Read the model definition and answer for the solid it produces. Units are mm, in the model's axes. Face numbers are marked on the shaded views. A direction names the side the tool comes from. Coordinates: 2 decimals unless noted, no trailing zeros. Loops run counter-clockwise (first coordinate to the right, second up) from the corner with the lowest first, then second, coordinate; pieces in that order, holes last. Notation, with made-up numbers: M -3.75,-20.5 L 37.25,-20.5 A34 cw 37.25,16.5 Z; hole C -1,-33.5 d7. An arc over 180 degrees is marked long. Put each result on its own line as item: value.
from build123d import *
from OCP.BRepFilletAPI import BRepFilletAPI_MakeChamfer

# Parameters (mm, degrees)
BOSS_EXTRUDE1_DEPTH = 15
CHAMFER1_SIZE       = 15
CHAMFER1_SIZE2      = 2
SKETCH2_R           = 3
CUT_EXTRUDE1_DEPTH  = 15
CHAMFER2_SIZE       = 2


with BuildPart() as part:
    # Sketch1 → Boss-Extrude1 (new body)
    with BuildSketch(Plane(origin=(0, 0, 0), x_dir=(1, 0, 0), z_dir=(0, 1, 0))):
        with BuildLine():
            ThreePointArc((-10, 0), (0, 10), (10, 0))
            Line((10, 0), (10, 25))
            Line((10, 25), (-10, 25))
            Line((-10, 25), (-10, 0))
        make_face()
        with BuildLine():
            ThreePointArc((-4.8, 0), (0, 4.8), (4.8, 0))
            Line((4.8, 0), (10, 0))
            ThreePointArc((10, 0), (0, 10), (-10, 0))
            Line((-10, 0), (-4.8, 0))
        make_face()
        with BuildLine():
            Line((10, 0), (4.8, 0))
            ThreePointArc((4.8, 0), (0, -4.8), (-4.8, 0))
            Line((-4.8, 0), (-10, 0))
            ThreePointArc((-10, 0), (0, -10), (10, 0))
        make_face()
    extrude(amount=BOSS_EXTRUDE1_DEPTH)

    # Chamfer1: one chamfer whose edges measure the first distance from different faces: ONE call of the kernel's chamfer builder (chamfer() names one face for all edges)
    chamfer1_edges_1 = [part.edges().sort_by_distance(p)[0] for p in [
        (-10, 7.5, -25),
    ]]
    chamfer1_side_1 = [part.faces().sort_by_distance(p)[0] for p in [
        (-10, 7.5, -12.5),
    ]]
    chamfer1_edges_2 = [part.edges().sort_by_distance(p)[0] for p in [
        (10, 7.5, -25),
    ]]
    chamfer1_side_2 = [part.faces().sort_by_distance(p)[0] for p in [
        (10, 7.5, -12.5),
    ]]
    chamfer1_edges_3 = [part.edges().sort_by_distance(p)[0] for p in [
        (0, 15, -25),
    ]]
    chamfer1_side_3 = [part.faces().sort_by_distance(p)[0] for p in [
        (0, 15, -9.549099972),
    ]]
    chamfer1 = BRepFilletAPI_MakeChamfer(part.part.solid().wrapped)
    for e in chamfer1_edges_1:
        chamfer1.Add(CHAMFER1_SIZE, CHAMFER1_SIZE2, e.wrapped, chamfer1_side_1[0].wrapped)  # the first distance lies on this face
    for e in chamfer1_edges_2:
        chamfer1.Add(CHAMFER1_SIZE, CHAMFER1_SIZE2, e.wrapped, chamfer1_side_2[0].wrapped)  # the first distance lies on this face
    for e in chamfer1_edges_3:
        chamfer1.Add(CHAMFER1_SIZE, CHAMFER1_SIZE2, e.wrapped, chamfer1_side_3[0].wrapped)  # the first distance lies on this face
    add(Compound.cast(chamfer1.Shape()), mode=Mode.REPLACE)

    # Sketch2 → Cut-Extrude1 (cut)
    with BuildSketch(Plane(origin=(0, 0, -25), x_dir=(-1, 0, 0), z_dir=(0, 0, -1))):
        with Locations((0, 7.2)):
            Circle(SKETCH2_R)
    extrude(amount=-CUT_EXTRUDE1_DEPTH, mode=Mode.SUBTRACT)

    # Chamfer2
    chamfer2_edges = [part.edges().sort_by_distance(p)[0] for p in [
        (0, 0, 10),
        (0, 15, 10),
        (-10, 15, -5),
        (-10, 0, -5),
        (10, 0, -5),
        (10, 15, -5),
    ]]
    chamfer(chamfer2_edges, length=CHAMFER2_SIZE)


solid = part.part
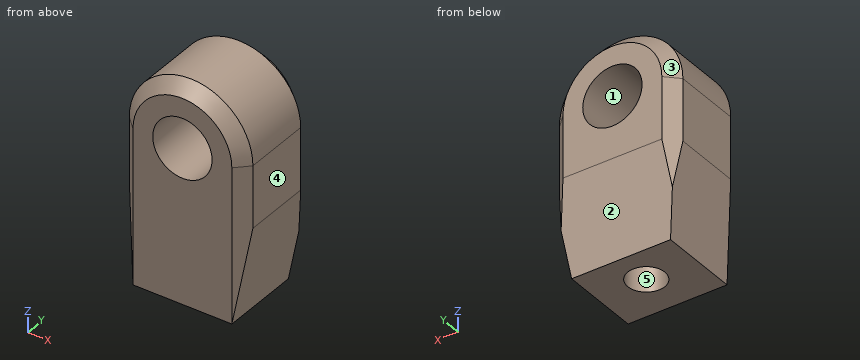
1) Which of the six approach directions +Z, -Z, +X, -X, +Y, -Y give full straight-line access (tool end or side, diameter ignored) to the marked faces 4 and 5?
Answer list:
face 4: +Z, -Z, +X, +Y, -Y
face 5: -Z
2) Determine the mould class of the marked faces 1, 2 and 3 for opening direction Z: released by +Z, released by -Z, zero draft, split by the parting line, or undercut.
Answer list:
face 1: undercut
face 2: released by -Z
face 3: released by +Z
3) Find section B-B, the plane y = 7.2. Write down the section's boundary in (x, z).
Answer list:
outline: M -10,-10 L -8,-25 L -3,-25 L -3,-10 L 3,-10 L 3,-25 L 8,-25 L 10,-10 L 10,0 A10 ccw -10,0 Z; hole C 0,0 d9.6
4) Find section A-A, the plane x = 0. Write down the section's boundary in (y, z).
Answer list:
outline: M 0,-25 L 4.2,-25 L 4.2,-10 L 10.2,-10 L 10.2,-25 L 13,-25 L 15,-10 L 15,-4.8 L 0,-4.8 Z; M 0,4.8 L 15,4.8 L 15,8 L 13,10 L 2,10 L 0,8 Z
5) Find section C-C, the plane z = -20. Write down the section's boundary in (x, y), plus the area to 3 significant figures.
Answer list:
outline: M -8.67,0.67 L -8,0 L 8,0 L 8.67,0.67 L 8.67,13.67 L -8.67,13.67 Z; hole C 0,7.2 d6
area: 208 mm^2
6) Given pin 1 Ø1 at (x, y) = (1.5, 7) entering from -Z; pin 2 Ø6 at (x, y) = (8, 2.5) entering from +Z; pin 3 Ø6 at (x, y) = (-4.5, 5) entering from +Z, each flat-ended and moving along its own axis, determine where each tip first touches the part or whether it passes through.
Answer list:
pin 1: stops at z = -10
pin 2: stops at z = 8.66
pin 3: stops at z = 9.89
7) Find section D-D, the plane z = -2.5. Write down the section's boundary in (x, y).
Answer list:
outline: M -10,2 L -8,0 L -4.1,0 L -4.1,15 L -8,15 L -10,13 Z; M 4.1,0 L 8,0 L 10,2 L 10,13 L 8,15 L 4.1,15 Z
8) Straight lines are drawn through the part: line 1 (Z direction, x = 0, y = 5.5); line 2 (X direction, y = 8.75, z = -1); line 3 (X direction, y = 9, z = -15.5). For each, find the intervals that lie inside material, in ascending order. Write a range as [from, to].
Answer list:
line 1: z = [-10, -4.8], [4.8, 10]
line 2: x = [-10, -4.69], [4.69, 10]
line 3: x = [-9.27, -2.4], [2.4, 9.27]
